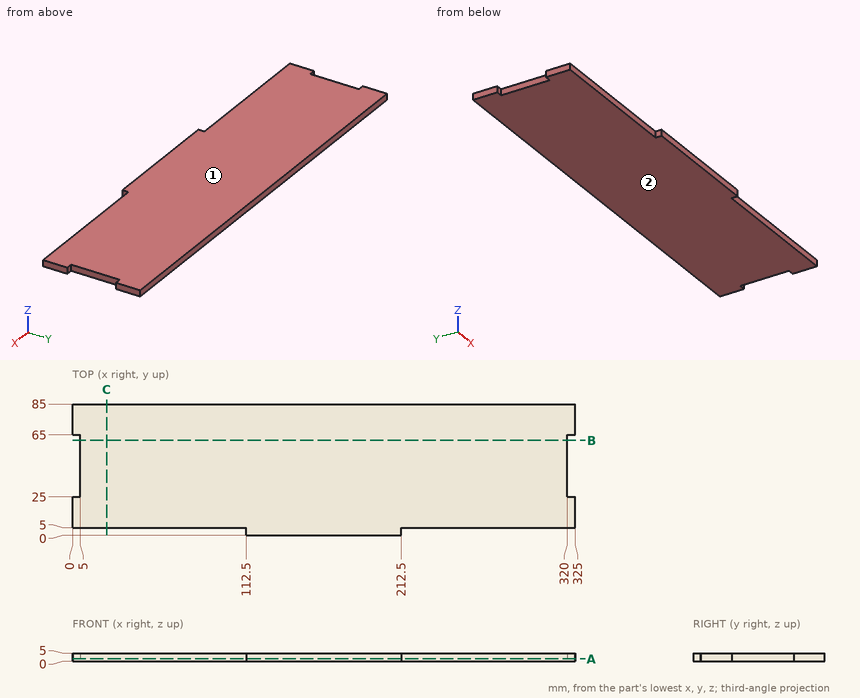
Design review of the part shown in the three views and the two pictorial views. Dimensions are in mm from the part's minimum x, y and z. Coordinates: 2 decimals unless noted, no trailing zeros. Write each loop counter-clockwise with the first axis right and the second up, starting at its lowest first coordinate (ties: lowest second). Pieces come first, ordered by that corner, then holes. Notation, with made-up numbers: (15, 14.25) -> (63, 14.25) arc R35 ccw to (63, 47.25) -> close; hole circle Ø8 at (-17.75, 30). An arc over 180 degrees is marked (long way). Answer in a Markdown table with one row per item.
1. Clearance check with flat-ended pins moving along their axes: pin 1 Ø6 at (x, y) = (134, 38) entering from -Z; pin 2 Ø1.5 at (x, z) = (35, 2) entering from -Y; pin 3 Ø1.5 at (y, z) = (38.5, 1.5) entering from -X; pin 4 Ø2.5 at (y, z) = (1.5, 3.5) entering from -X. State where each tip first meets the part, or that it passes through.
Answers below:
| item | result |
|---|---|
| pin 1 | stops at z = 0 |
| pin 2 | stops at y = 5 |
| pin 3 | stops at x = 5 |
| pin 4 | stops at x = 112.5 |
2. Wall thickness on probe 1 along Y at (x, z) = (93, 4); probe 2 along X at (y, z) = (37.5, 4.2): over which ranges is each line inside the solid? List them lowest first. Write a range as [from, to].
Answers below:
| item | result |
|---|---|
| probe 1 | y = [5, 85] |
| probe 2 | x = [5, 320] |
3. We need section C-C, the plane x = 22. State the section outline as (y, z) points.
Answers below:
| item | result |
|---|---|
| outline | (5, 0) -> (85, 0) -> (85, 5) -> (5, 5) -> close |
4. Draft analysis for pull direction Z (two halves, no side actions). For the marked faces 1 and 2, state which applies: +Z half, -Z half, draft (parallel to the pull), parting line (faces both ways), or undercut.
Answers below:
| item | result |
|---|---|
| face 1 | +Z half |
| face 2 | -Z half |
5. We need section B-B, the plane y = 61.5. State the section outline as (x, z) points.
Answers below:
| item | result |
|---|---|
| outline | (5, 0) -> (320, 0) -> (320, 5) -> (5, 5) -> close |
6. We need section A-A, the plane z = 1.5. State the section outline as (x, y) points, and give its area (3 significant figures).
Answers below:
| item | result |
|---|---|
| outline | (0, 5) -> (112.5, 5) -> (112.5, 0) -> (212.5, 0) -> (212.5, 5) -> (325, 5) -> (325, 25) -> (320, 25) -> (320, 65) -> (325, 65) -> (325, 85) -> (0, 85) -> (0, 65) -> (5, 65) -> (5, 25) -> (0, 25) -> close |
| area | 26,100 mm^2 |
